Verification items for the finished model (mm, model axes). Face numbers are marked on the shaded views. A direction names the side the tool comes from. Give positions to 0.01 mm unless a question says otherwise; leave off trailing zeros. Order: outer loops, then holes, each group sorted by start corner. A loop starts at its lowest first (then second) coordinate and runs counter-clockwise, first axis right, second up. Notation, with made-up numbers: (11.5, -1.75) -> (62.5, -1.75) arc R15 ccw to (62.5, 20.25) -> close; hole circle Ø10 at (-29, 45). An arc over 180 degrees is marked (long way). Return JSON: item names as keys, results as strings. Group by question number.
(1) Thickness scan on line 1 along Z through (x, y) = (-6, 23.5); line 2 along Z through (x, y) = (-1, 76); line 3 along X through (y, z) = (42, 29.5). Record the ranges inside material, lowest first.
(2) Tool access check on the marked faces 1, 2, 3, 4 and 5. Record the directions out of +Z, -Z, +X, -X, +Y, -Y that give a thin tool (end or side, any length) a straight path to the whole face; none if there is none.
(3) Cross-section at C-C on y = 32.5. Enter the section's corners in (x, z).
(4) Depth check by flat-ended pin: pin 1 Ø6 at (x, z) = (-17.5, -9.5) entering from +Y; pin 2 Ø1.5 at (y, z) = (69, -12.5) entering from -X; pin 3 Ø3 at (x, z) = (-6, 3.5) entering from -Y. Enter the tip coordinate at first touch or a pass-through.
(5) Cross-section at D-D on z = 39. Enter the section's corners in (x, y), then the cut area to 3 significant figures.
(6) Cross-section at B-B on z = -13. Enter the section's corners in (x, y), then the cut area to 3 significant figures.
(7) Cross-section at A-A on y = 74. Enter the section's corners in (x, z).
(8) Release check for a two-part mould opening along Z. For the marked faces 6, 7, 8 and 9 record: pulls with the +Z half, pulls with the -Z half, needs draft (parallel to the pull), parting line crosses it, or undercut.
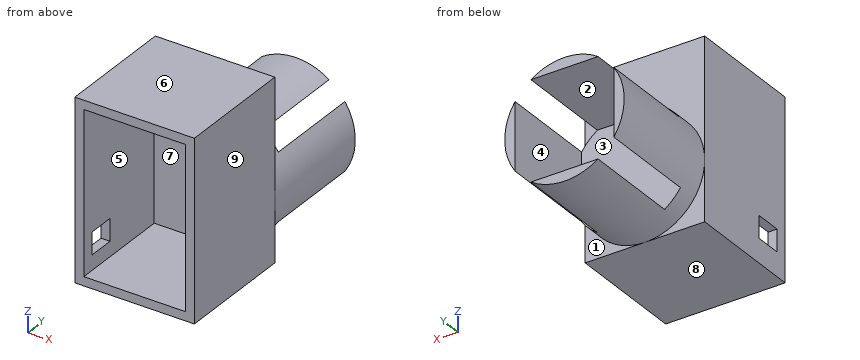
from build123d import *

# Parameters (mm, degrees)
SKETCH1_R           = 25.4
BOSS_EXTRUDE1_DEPTH = 101.6
SKETCH2_W           = 42.0116
SKETCH2_H           = 42.0116
CUT_EXTRUDE1_DEPTH  = 42.0116
SKETCH3_W           = 50.8
SKETCH3_H           = 76.2
BOSS_EXTRUDE2_DEPTH = 50.8
SKETCH4_W           = 43.18
SKETCH4_H           = 68.58
CUT_EXTRUDE2_DEPTH  = 44.45
CUT_EXTRUDE3_REACH  = 126.434
SKETCH5_W           = 9.398
SKETCH5_H           = 11.43


with BuildPart() as part:
    # Sketch1 → Boss-Extrude1 (new body)
    with BuildSketch(Plane(origin=(0, 0, 0), x_dir=(1, 0, 0), z_dir=(0, 1, 0))):
        with Locations(Location((0, 0, 0), (0, 0, 270))):
            Circle(SKETCH1_R)
    extrude(amount=BOSS_EXTRUDE1_DEPTH)

    # Sketch2 → Cut-Extrude1 (cut)
    with BuildSketch(Plane(origin=(0, 101.6, 0), x_dir=(1, 0, 0), z_dir=(0, 1, 0))):
        Rectangle(SKETCH2_W, SKETCH2_H)
    extrude(amount=-CUT_EXTRUDE1_DEPTH, mode=Mode.SUBTRACT)

    # Sketch3 → Boss-Extrude2 (add)
    with BuildSketch(Plane.XZ):
        with Locations((0, 12.7)):
            Rectangle(SKETCH3_W, SKETCH3_H)
    extrude(amount=-BOSS_EXTRUDE2_DEPTH)

    # Sketch4 → Cut-Extrude2 (cut)
    with BuildSketch(Plane.XZ):
        with Locations((0, 12.7)):
            Rectangle(SKETCH4_W, SKETCH4_H)
    extrude(amount=-CUT_EXTRUDE2_DEPTH, mode=Mode.SUBTRACT)

    # Sketch5 → Cut-Extrude3 (cut, up to next)
    with BuildSketch(Plane.ZY.offset(25.4), mode=Mode.PRIVATE) as cut_extrude3_sk1:
        with Locations((-10.541, 10.795)):
            Rectangle(SKETCH5_W, SKETCH5_H)
    cut_extrude3_tool1 = extrude(cut_extrude3_sk1.sketch, amount=-CUT_EXTRUDE3_REACH, mode=Mode.PRIVATE) & part.part
    add(cut_extrude3_tool1.solids().sort_by_distance((-25.4, 10.795, -10.541))[0], mode=Mode.SUBTRACT)


solid = part.part
Verdict:
{
 "1": {"line 1": "-25.4 to -21.59, 46.99 to 50.8", "line 2": "-25.38 to -21.01, 21.01 to 25.38", "line 3": "-25.4 to -21.59, 21.59 to 25.4"},
 "2": {"face 1": "-Z, +X, +Y", "face 2": "+X, -X, +Y", "face 3": "+Y", "face 4": "+Z, -Z, +Y", "face 5": "-Y"},
 "3": {"outline": "(-25.4, -25.4) -> (25.4, -25.4) -> (25.4, 50.8) -> (-25.4, 50.8) -> close; hole (-21.59, -21.59) -> (21.59, -21.59) -> (21.59, 46.99) -> (-21.59, 46.99) -> close"},
 "4": {"pin 1": "y = 59.59", "pin 2": "x = -22.52", "pin 3": "y = 44.45"},
 "5": {"outline": "(-25.4, 0) -> (-21.59, 0) -> (-21.59, 44.45) -> (21.59, 44.45) -> (21.59, 0) -> (25.4, 0) -> (25.4, 50.8) -> (-25.4, 50.8) -> close", "area": "661 mm²"},
 "6": {"outline": "(-25.4, 0) -> (-21.59, 0) -> (-21.59, 5.08) -> (-25.4, 5.08) -> close; (-25.4, 16.51) -> (-21.59, 16.51) -> (-21.59, 44.45) -> (21.59, 44.45) -> (21.59, 0) -> (25.4, 0) -> (25.4, 50.8) -> (21.82, 50.8) -> (21.82, 101.6) -> (21.01, 101.6) -> (21.01, 59.59) -> (-21.01, 59.59) -> (-21.01, 101.6) -> (-21.82, 101.6) -> (-21.82, 50.8) -> (-25.4, 50.8) -> close", "area": "1,070 mm²"},
 "7": {"outline": "(-21.01, -14.28) -> (-21.01, 14.28) arc R25.4 ccw to start; (-14.28, -21.01) arc R25.4 ccw to (14.28, -21.01) -> close; (-14.28, 21.01) -> (14.28, 21.01) arc R25.4 ccw to start; (21.01, -14.28) arc R25.4 ccw to (21.01, 14.28) -> close"},
 "8": {"face 6": "pulls with the +Z half", "face 7": "undercut", "face 8": "pulls with the -Z half", "face 9": "needs draft"}
}
